Source: CAD feature listing. Evaluate the final solid. Frame: model axes, mm. Face numbers are marked on the shaded views. A direction names the side the tool comes from. Coordinates: 2 decimals unless noted, no trailing zeros. Loops run counter-clockwise (first coordinate to the right, second up) from the corner with the lowest first, then second, coordinate; pieces in that order, holes last.
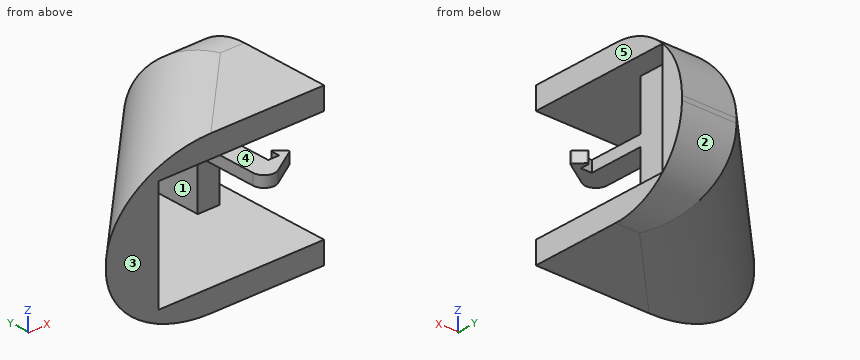
```python
from build123d import *

# Parameters (mm, degrees)
BOSS_EXTRUDE1_DEPTH = 7
SHELL1_T            = -2
BOSS_EXTRUDE2_REACH = 14
SKETCH2_W           = 2
SKETCH2_H           = 10
SKETCH3_W           = 2
SKETCH3_H           = 1
BOSS_EXTRUDE3_DEPTH = 5
SKETCH4_W           = 15.171572875
SKETCH4_H           = 10
CUT_EXTRUDE1_DEPTH  = 5
SKETCH5_W           = 4
SKETCH5_H           = 1
BOSS_EXTRUDE4_DEPTH = 2.5
CUT_EXTRUDE2_REACH  = 9.5
BOSS_EXTRUDE5_START = -1
BOSS_EXTRUDE5_DEPTH = 1
FILLET2_R           = 0.1
FILLET3_R           = 1
FILLET4_R           = 6.8


with BuildPart() as part:
    # Sketch1 → Boss-Extrude1 (new body, symmetric)
    with BuildSketch(Plane.XY):
        Polygon((0, 0), (0, 15), (-5, 15), (-20, 0), align=None)
    extrude(amount=BOSS_EXTRUDE1_DEPTH, both=True)

    # Shell1
    shell1_openings = [part.faces().sort_by_distance(p)[0] for p in [
        (0, 7.5, 0),
    ]]
    offset(amount=SHELL1_T, openings=shell1_openings, kind=Kind.INTERSECTION)

    # Sketch2 → Boss-Extrude2 (add, up to next)
    with BuildSketch(Plane.XY.offset(-5), mode=Mode.PRIVATE) as boss_extrude2_sk1:
        with Locations((-3, 13.501498051)):
            Rectangle(SKETCH2_W, SKETCH2_H)
    boss_extrude2_tool1 = extrude(boss_extrude2_sk1.sketch, amount=BOSS_EXTRUDE2_REACH, mode=Mode.PRIVATE) - part.part
    add(boss_extrude2_tool1.solids().sort_by_distance((-3, 13.501498, -5))[0])

    # Sketch3 → Boss-Extrude3 (add)
    with BuildSketch(Plane.XZ.offset(-8.501498051)):
        with Locations((-3, 0)):
            Rectangle(SKETCH3_W, SKETCH3_H)
    extrude(amount=BOSS_EXTRUDE3_DEPTH)

    # Sketch4 → Cut-Extrude1 (cut)
    with BuildSketch(Plane(origin=(0, 2, 0), x_dir=(1, 0, 0), z_dir=(0, 1, 0))):
        with Locations((-7.585786438, 0)):
            Rectangle(SKETCH4_W, SKETCH4_H)
    extrude(amount=-CUT_EXTRUDE1_DEPTH, mode=Mode.SUBTRACT)

    # Sketch5 → Boss-Extrude4 (add)
    with BuildSketch(Plane(origin=(0, 3.501498051, 0), x_dir=(-1, 0, 0), z_dir=(0, -1, 0))):
        with Locations((2, 0)):
            Rectangle(SKETCH5_W, SKETCH5_H)
    extrude(amount=BOSS_EXTRUDE4_DEPTH)

    # Sketch6 → Cut-Extrude2 (cut, up to next)
    with BuildSketch(Plane.XY.offset(0.5), mode=Mode.PRIVATE) as cut_extrude2_sk1:
        Polygon((0, 3.501498051), (-4, 1.001498051), (0, 1.001498051), align=None)
    cut_extrude2_tool1 = extrude(cut_extrude2_sk1.sketch, amount=-CUT_EXTRUDE2_REACH, mode=Mode.PRIVATE) & part.part
    add(cut_extrude2_tool1.solids().sort_by_distance((-1.333333, 1.834831, 0.5))[0], mode=Mode.SUBTRACT)

    # Sketch7 → Boss-Extrude5 (add)
    with BuildSketch(Plane.XY.offset(0.5).offset(BOSS_EXTRUDE5_START)):
        Polygon((0, 3.501498051), (-1, 3.501498051), (-1, 4.501498051), align=None)
    extrude(amount=BOSS_EXTRUDE5_DEPTH)

    # Fillet2
    fillet2_edges = [part.edges().sort_by_distance(p)[0] for p in [
        (0, 3.501498051, 0),
        (-1, 4.501498051, 0),
    ]]
    fillet(fillet2_edges, radius=FILLET2_R)

    # Fillet3
    fillet3_edges = [part.edges().sort_by_distance(p)[0] for p in [
        (-4, 1.001498051, 0),
    ]]
    fillet(fillet3_edges, radius=FILLET3_R)

    # Fillet4
    fillet4_edges = [part.edges().sort_by_distance(p)[0] for p in [
        (-2.5, 15, 7),
        (-12.5, 7.5, 7),
        (-12.5, 7.5, -7),
        (-2.5, 15, -7),
    ]]
    fillet(fillet4_edges, radius=FILLET4_R)


solid = part.part
```
Q1. Draft query along Z for the marked faces 1, 2 and 3. Return one class per face: released by +Z, released by -Z, zero draft, split by the parting line, or undercut.
Q2. Section query A-A on x = -1.75. Return the cut outline in (y, z), then the cut area to 3 significant figures.
Q3. Material intervals for line 1 along Z through (x, y) = (-3, 2.25); line 2 along Z through (x, y) = (-1.5, 7.75); line 3 along X through (y, z) = (11.75, -3.75), sorted ascending.
Q4. Reachability of the marked faces 4 and 5 from +Z, -Z, +X, -X, +Y, -Y: full face, straight path, thin tool, end or side. Return the list, or none.
Q5. Section query C-C on z = 1.75. Return the cut outline in (x, y).
Q6. First-contact query: pin 1 Ø3 at (x, z) = (-9, -2) entering from -Y; pin 2 Ø0.6 at (y, z) = (1, -2) entering from +X; pin 3 Ø0.6 at (x, z) = (-2.5, 3) entering from -Y. Flat tips, straight axial feed; report the tip coordinate or a pass-through.
Q7. Section query B-B on z = 3.25. Return the cut outline in (x, y).
Q8. Section query D-D on z = 6. Return the cut outline in (x, y).
Resolved:
1. face 1: undercut
1. face 2: released by -Z
1. face 3: zero draft
2. outline: (0, -7) - (8.2, -7) arc R6.8 ccw to (15, -0.2) - (15, 0.2) arc R6.8 ccw to (8.2, 7) - (0, 7) - (0, 5) - (13, 5) - (13, -5) - (0, -5) - close; (2.41, -0.5) - (3.5, -0.5) - (3.5, 0.5) - (2.41, 0.5) - close
2. area: 61.2 mm2
3. line 1: z = -7 to -5, -0.5 to 0.5, 5 to 7
3. line 2: z = -7 to -5, 5 to 7
3. line 3: x = -6.84 to -5.42, -4 to -2
4. face 4: +X, -Y
4. face 5: +Z, -Z, +X, +Y, -Y
5. outline: (-19.75, 0) - (-15.17, 0) - (-15.17, 2) - (-4.17, 13) - (-4, 13) - (-4, 8.5) - (-2, 8.5) - (-2, 13) - (0, 13) - (0, 14.82) - (-4.93, 14.82) - close
6. pin 1: stops at y = 6.67
6. pin 2: stops at x = -15.17
6. pin 3: stops at y = 8.5
7. outline: (-18.98, 0) - (-15.17, 0) - (-15.17, 2) - (-4.17, 13) - (-4, 13) - (-4, 8.5) - (-2, 8.5) - (-2, 13) - (0, 13) - (0, 14.28) - (-4.7, 14.28) - close
8. outline: (-15.4, 0) - (0, 0) - (0, 11.75) - (-3.65, 11.75) - close
